The figure shows three views and two pictorial views of one solid part (mm, origin at its lowest corner). Answer the questions. A direction names the side the tool comes from. Coordinates: 2 decimals unless noted, no trailing zeros. Order: outer loops, then holes, each group sorted by start corner. A loop starts at its lowest first (then second) coordinate and runs counter-clockwise, first axis right, second up. Notation, with made-up numbers: (-5, -23) - (40, -23) arc R14 cw to (40, -12) - close; hole circle Ø6 at (73.5, -39). An arc over 180 degrees is marked (long way). Use one line per item in the form item = value. Start each with the question number.
Item 1: Section B-B, the plane y = 6 is taken. Write down the section's boundary in (x, z), and give its area (3 significant figures).
Item 2: Section A-A, the plane z = 1.75 is taken. Write down the section's boundary in (x, y).
Item 3: Each of these flat-tipped pins is pushed along its axis until it touches: pin 1 Ø2.5 at (y, z) = (35, 5) entering from +X; pin 2 Ø4 at (x, z) = (27, 3) entering from +Y; pin 3 Ø4 at (y, z) = (59, 4.5) entering from -X. Where does it stop, or does it pass through?
Item 4: Consider line 1 along X through (y, z) = (60, 1.25); line 2 along Y through (x, z) = (26, 6); line 3 along Y through (x, z) = (29, 2.5). Determine where each line is inside the solid, lowest interval first. Write a range as [from, to].
Item 5: A tool of negligible diameter and unlimited length cuts with its end or side. For the marked faces 1, 2 and 3, from which of +Z, -Z, +X, -X, +Y, -Y can it reach the whole face along a straight path? Write none if from no direction.
Item 6: Section C-C, the plane x = 19.5 is taken. Write down the section's boundary in (y, z), and give its area (3 significant figures).
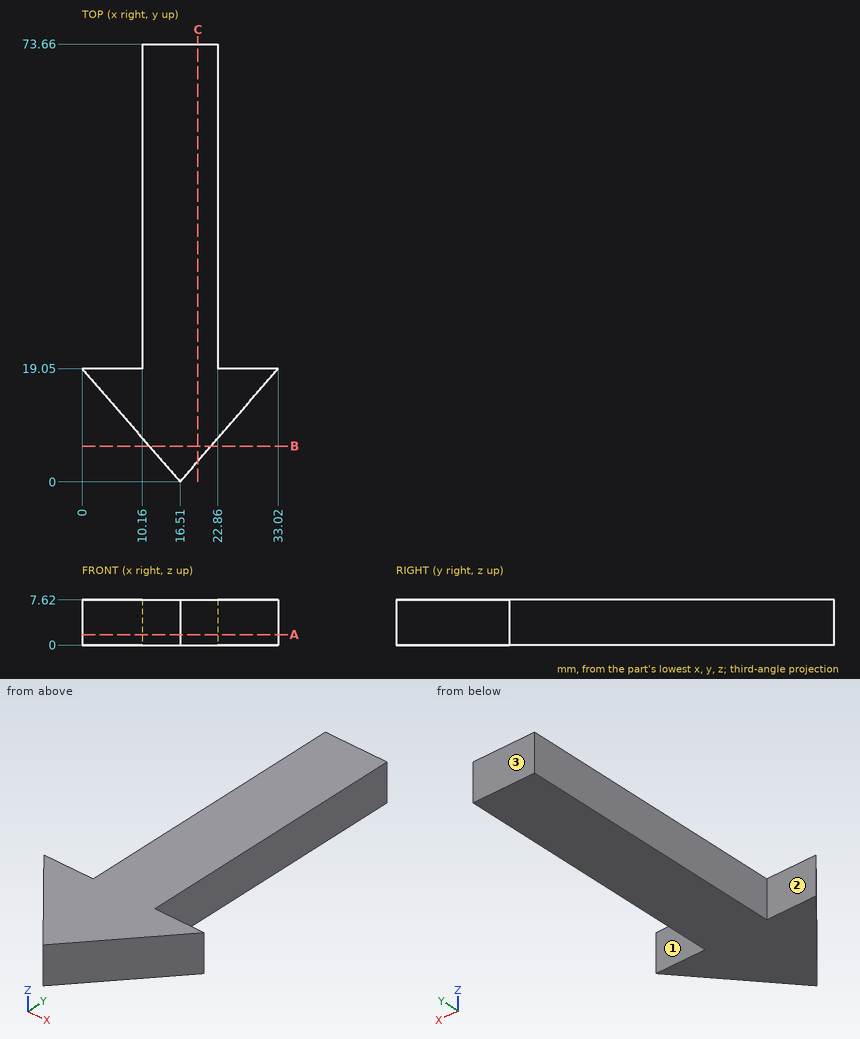
Response:
q1.outline = (11.31, 0) - (21.71, 0) - (21.71, 7.62) - (11.31, 7.62) - close
q1.area = 79.2 mm2
q2.outline = (0, 19.05) - (16.51, 0) - (33.02, 19.05) - (22.86, 19.05) - (22.86, 73.66) - (10.16, 73.66) - (10.16, 19.05) - close
q3.pin_1 = 22.86
q3.pin_2 = 19.05
q3.pin_3 = 10.16
q4.line_1 = [10.16, 22.86]
q4.line_2 = [10.95, 19.05]
q4.line_3 = [14.41, 19.05]
q5.face_1 = +Z, -Z, +X, +Y
q5.face_2 = +Z, -Z, -X, +Y
q5.face_3 = +Z, -Z, +X, -X, +Y
q6.outline = (3.45, 0) - (73.66, 0) - (73.66, 7.62) - (3.45, 7.62) - close
q6.area = 535 mm2
